Source: CAD feature listing. Evaluate the final solid. Frame: model axes, mm. Give positions to 0.01 mm unless a question says otherwise; leave off trailing zeros. Write each loop counter-clockwise with the first axis right and the second up, starting at its lowest first coordinate (ties: lowest second). Pieces come first, ordered by that corner, then holes. Notation, with made-up numbers: (26.25, 3.25) - (58.25, 3.25) arc R28 ccw to (58.25, 30.25) - close; hole circle Ø2 at (60.5, 86.25). An arc over 180 degrees is marked (long way). One line per question, with ' | ' between items. Start each with the question number.
(1) Section A-A, the plane y = 38.5. Return loops of the section in (x, z).
(2) Section B-B, the plane x = 25. Return loops of the section in (y, z).
(3) Ray query, line 1 (Z direction, x = -196.5, y = 27); line 2 (Z direction, x = -186, y = 7.5); line 3 (Z direction, x = 117, y = 41). Return the intervals inside material, ascending. Write a range as [from, to].
(4) Pin query (flat end, axial travel): pin 1 (1.5 mm diameter, centred on x = -125, y = 38, fed in from -Z); pin 2 (5 mm diameter, centred on x = -138, y = 27.5, fed in from -Z); pin 3 (6 mm diameter, centred on y = 21, z = 122.5, fed in from +X). Return the tip coordinate at first contact, or that it passes through.
(5) Section C-C, the plane z = 26.5. Return loops of the section in (x, y).
(6) Draft query along Z for faces 1 (the flat face through (99, 25, 219.55)), 2 (the cylindrical face through (-191.34, 24.65, 107.66)), 3 (the flat face through (-300, 25, 103)). Return one class per face: +Z half, -Z half, draft (parallel to the pull), parting line (faces both ways), or undercut.
Autodesk Inventor part; units mm, degrees
ref_plane "YZ Plane" through (0, 0, 0) normal (1, 0, 0) x (0, 1, 0)
ref_plane "XZ Plane" through (0, 0, 0) normal (0, 1, 0) x (-1, 0, 0)
ref_plane "XY Plane" through (0, 0, 0) normal (0, 0, 1) x (1, 0, 0)
sketch "Sketch1" plane through (0, 0, 0) normal (0, 1, 0) x (-1, 0, 0)
  line L0 (0, -151.455) -> (0, 151.455) construction
  line L1 (30.6851, 0) -> (-30.6851, 0) construction
  arc A0 (184.1467, -119.55) -> (0, 219.55) centre (0, 0) ccw
  line L2 (0, 219.55) -> (-200, 219.55)
  line L3 (-200, 219.55) -> (-200, 319.55)
  line L4 (-200, 319.55) -> (300, 319.55)
  line L5 (300, 319.55) -> (300, -119.55)
  line L6 (300, -119.55) -> (184.1467, -119.55)
  dimension "d0" = 439.1
  dimension "d1" = 200
  dimension "d3" = 100
  dimension "d4" = 119.55
  dimension "d5" = 300
extrude "Extrusion1" add sketch "Sketch1" along normal blind 50
properties part number "WoodBoundaryV1"
Check sheet entries:
1) outline: (-300, -119.55) - (-184.15, -119.55) arc R219.55 cw to (0, 219.55) - (200, 219.55) - (200, 319.55) - (-300, 319.55) - close
2) outline: (0, 219.55) - (50, 219.55) - (50, 319.55) - (0, 319.55) - close
3) line 1: [-119.55, -97.93], [97.93, 319.55] | line 2: [-119.55, -116.65], [116.65, 319.55] | line 3: [219.55, 319.55]
4) pin 1: z = 179.97 | pin 2: z = 168.71 | pin 3: x = -180.14
5) outline: (-300, 0) - (-217.94, 0) - (-217.94, 50) - (-300, 50) - close
6) face 1: -Z half | face 2: undercut | face 3: draft
